Work out the finished part from the listing and answer in its coordinate system (mm). Face numbers are marked on the shaded views. A direction names the side the tool comes from. Give positions to 0.01 mm unless a question says otherwise; leave off trailing zeros. Loops run counter-clockwise (first coordinate to the right, second up) from the corner with the lowest first, then second, coordinate; pieces in that order, holes last. Notation, with made-up numbers: M -19,27.5 L 11,27.5 A27 cw 11,61.5 Z; hole C 9.5,60 d11. An arc over 180 degrees is marked long. Write item = value, one per line. Start each with the question number.
1. Section A-A on x = 18 is taken. Determine the outline of the cut face in (y, z), plus the area to 3 significant figures.
2. Consider L1, parallel to Y at x = 5.5, z = 1.6. Determine where the line is inside the solid, lowest interval first. Write a range as [from, to].
3. Section B-B on y = 2.85 is taken. Give the number of separate pieces and of enclosed holes in the cut face, plus the area to 3 significant figures.
4. A flat-ended cylindrical pin translates along its axis: pin 1 Ø0.5 at (x, z) = (2.5, 1.5) entering from +Y. Find the tip coordinate at first contact, or state that the pin passes through.
5. For the marked faces 1 and 2, determine the directions among +Z, -Z, +X, -X, +Y, -Y from which every point of the face is accessible in a straight line to the end or side of a thin tool.
```python
from build123d import *

# Parameters (mm, degrees)
SKETCH3_W           = 30
SKETCH3_H           = 1
BOSS_EXTRUDE1_DEPTH = 5
BOSS_EXTRUDE2_DEPTH = 5
LPATTERN1_COUNT     = 10
LPATTERN1_PITCH     = 3.1


with BuildPart() as part:
    # Sketch3 → Boss-Extrude1 (new body)
    with BuildSketch(Plane.XY):
        with Locations((15, 0.5)):
            Rectangle(SKETCH3_W, SKETCH3_H)
    extrude(amount=BOSS_EXTRUDE1_DEPTH)

    # Sketch5 → Boss-Extrude2 (add)
    with BuildSketch(Plane.XY.offset(5)):
        Polygon((0, 1), (0.55, 5.92), (1.55, 5.92), (2.1, 1), align=None)
    boss_extrude2 = extrude(amount=-BOSS_EXTRUDE2_DEPTH)

    # LPattern1: Boss-Extrude2 ×10
    with Locations(*[(i * LPATTERN1_PITCH, 0, 0) for i in range(1, LPATTERN1_COUNT)]):
        add(boss_extrude2)


solid = part.part
```
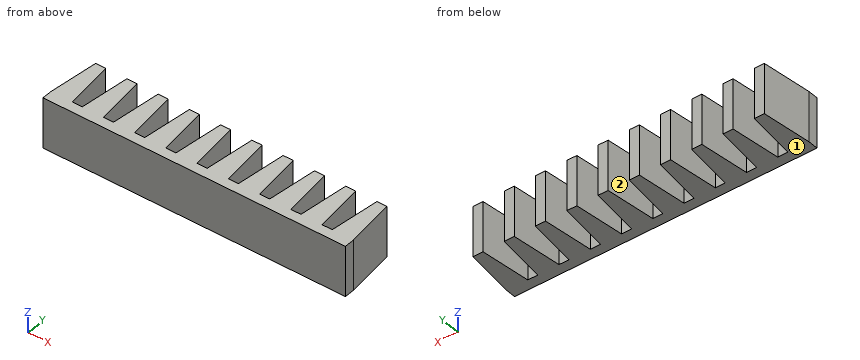
Verdict:
q1.outline = M 0,0 L 1,0 L 1,5 L 0,5 Z
q1.area = 5.00 mm2
q2.L1 = [0, 1]
q3.separate_pieces = 10
q3.enclosed_holes = 0
q3.area = 84.3 mm2
q4.pin_1 = 1
q5.face_1 = -Z, +X, -X, +Y, -Y
q5.face_2 = +Z, -Z, +Y
